Here's how the part is built. I have some questions about the finished solid (model axes, mm). A direction names the side the tool comes from. Give positions to 0.01 mm unless a question says otherwise; leave off trailing zeros. Write each loop counter-clockwise with the first axis right and the second up, starting at its lowest first coordinate (ties: lowest second). Pieces come first, ordered by that corner, then holes. Notation, with made-up numbers: (-9.75, 58) - (46.25, 58) arc R18 ccw to (46.25, 68) - close; hole circle Ø11 at (0, 55.5). An arc over 180 degrees is marked (long way). Use a Markdown table: item, result.
```python
from build123d import *

# Parameters (mm, degrees)
F1_DEPTH = 2
F2_R     = 1
F3_DEPTH = 2.001


with BuildPart() as f1:
    # F0 (on Top) → F1 (new body)
    with BuildSketch(Plane.XY):
        with BuildLine():
            ThreePointArc((7.271564, -1.836943), (7.442672, -0.925546), (7.5, 0))
            ThreePointArc((7.5, 0), (7.442672, 0.925546), (7.271564, 1.836943))
            ThreePointArc((7.271564, 1.836943), (7.132924, 2.317627), (6.962547, 2.788))
            ThreePointArc((6.962547, 2.788), (6.067627, 4.408389), (4.803091, 5.760236))
            ThreePointArc((4.803091, 5.760236), (4.408389, 6.067627), (3.994074, 6.348021))
            ThreePointArc((3.994074, 6.348021), (2.317627, 7.132924), (0.5, 7.483315))
            ThreePointArc((0.5, 7.483315), (0, 7.5), (-0.5, 7.483315))
            ThreePointArc((-0.5, 7.483315), (-2.317627, 7.132924), (-3.994074, 6.348021))
            ThreePointArc((-3.994074, 6.348021), (-4.408389, 6.067627), (-4.803091, 5.760236))
            ThreePointArc((-4.803091, 5.760236), (-6.067627, 4.408389), (-6.962547, 2.788))
            ThreePointArc((-6.962547, 2.788), (-7.132924, 2.317627), (-7.271564, 1.836943))
            ThreePointArc((-7.271564, 1.836943), (-7.5, 0), (-7.271564, -1.836943))
            ThreePointArc((-7.271564, -1.836943), (-7.132924, -2.317627), (-6.962547, -2.788))
            ThreePointArc((-6.962547, -2.788), (-6.067627, -4.408389), (-4.803091, -5.760236))
            ThreePointArc((-4.803091, -5.760236), (-4.408389, -6.067627), (-3.994074, -6.348021))
            ThreePointArc((-3.994074, -6.348021), (-2.317627, -7.132924), (-0.5, -7.483315))
            ThreePointArc((-0.5, -7.483315), (0, -7.5), (0.5, -7.483315))
            ThreePointArc((0.5, -7.483315), (2.317627, -7.132924), (3.994074, -6.348021))
            ThreePointArc((3.994074, -6.348021), (4.408389, -6.067627), (4.803091, -5.760236))
            ThreePointArc((4.803091, -5.760236), (6.067627, -4.408389), (6.962547, -2.788))
            ThreePointArc((6.962547, -2.788), (7.132924, -2.317627), (7.271564, -1.836943))
        make_face()
        with BuildLine():
            ThreePointArc((6.962547, 2.788), (7.132924, 2.317627), (7.271564, 1.836943))
            Line((7.271564, 1.836943), (9.189545, 2.460133))
            Line((9.189545, 2.460133), (9.035037, 2.935661))
            Line((9.035037, 2.935661), (8.880528, 3.41119))
            Line((8.880528, 3.41119), (6.962547, 2.788))
        make_face()
        with BuildLine():
            Line((9.189545, -2.460133), (7.271564, -1.836943))
            ThreePointArc((7.271564, -1.836943), (7.132924, -2.317627), (6.962547, -2.788))
            Line((6.962547, -2.788), (8.880528, -3.41119))
            Line((8.880528, -3.41119), (9.035037, -2.935661))
            Line((9.035037, -2.935661), (9.189545, -2.460133))
        make_face()
        with BuildLine():
            ThreePointArc((3.994074, 6.348021), (4.408389, 6.067627), (4.803091, 5.760236))
            Line((4.803091, 5.760236), (5.988468, 7.391769))
            Line((5.988468, 7.391769), (5.58396, 7.685661))
            Line((5.58396, 7.685661), (5.179451, 7.979554))
            Line((5.179451, 7.979554), (3.994074, 6.348021))
        make_face()
        with BuildLine():
            Line((5.988468, -7.391769), (4.803091, -5.760236))
            ThreePointArc((4.803091, -5.760236), (4.408389, -6.067627), (3.994074, -6.348021))
            Line((3.994074, -6.348021), (5.179451, -7.979554))
            Line((5.179451, -7.979554), (5.58396, -7.685661))
            Line((5.58396, -7.685661), (5.988468, -7.391769))
        make_face()
        with BuildLine():
            ThreePointArc((-0.5, 7.483315), (0, 7.5), (0.5, 7.483315))
            Line((0.5, 7.483315), (0.5, 9.5))
            Line((0.5, 9.5), (0, 9.5))
            Line((0, 9.5), (-0.5, 9.5))
            Line((-0.5, 9.5), (-0.5, 7.483315))
        make_face()
        with BuildLine():
            Line((0.5, -9.5), (0.5, -7.483315))
            ThreePointArc((0.5, -7.483315), (0, -7.5), (-0.5, -7.483315))
            Line((-0.5, -7.483315), (-0.5, -9.5))
            Line((-0.5, -9.5), (0, -9.5))
            Line((0, -9.5), (0.5, -9.5))
        make_face()
        with BuildLine():
            ThreePointArc((-4.803091, 5.760236), (-4.408389, 6.067627), (-3.994074, 6.348021))
            Line((-3.994074, 6.348021), (-5.179451, 7.979554))
            Line((-5.179451, 7.979554), (-5.58396, 7.685661))
            Line((-5.58396, 7.685661), (-5.988468, 7.391769))
            Line((-5.988468, 7.391769), (-4.803091, 5.760236))
        make_face()
        with BuildLine():
            Line((-5.179451, -7.979554), (-3.994074, -6.348021))
            ThreePointArc((-3.994074, -6.348021), (-4.408389, -6.067627), (-4.803091, -5.760236))
            Line((-4.803091, -5.760236), (-5.988468, -7.391769))
            Line((-5.988468, -7.391769), (-5.58396, -7.685661))
            Line((-5.58396, -7.685661), (-5.179451, -7.979554))
        make_face()
        with BuildLine():
            ThreePointArc((-7.271564, 1.836943), (-7.132924, 2.317627), (-6.962547, 2.788))
            Line((-6.962547, 2.788), (-8.880528, 3.41119))
            Line((-8.880528, 3.41119), (-9.035037, 2.935661))
            Line((-9.035037, 2.935661), (-9.189545, 2.460133))
            Line((-9.189545, 2.460133), (-7.271564, 1.836943))
        make_face()
        with BuildLine():
            Line((-8.880528, -3.41119), (-6.962547, -2.788))
            ThreePointArc((-6.962547, -2.788), (-7.132924, -2.317627), (-7.271564, -1.836943))
            Line((-7.271564, -1.836943), (-9.189545, -2.460133))
            Line((-9.189545, -2.460133), (-9.035037, -2.935661))
            Line((-9.035037, -2.935661), (-8.880528, -3.41119))
        make_face()
    extrude(amount=F1_DEPTH)

    # F2 (on face) → F3 (cut, through all)
    with BuildSketch(Plane.XY.offset(2)):
        Circle(F2_R)
    extrude(amount=-F3_DEPTH, mode=Mode.SUBTRACT)


solid = f1.part
```
Item 1: Thinking about a two-plate mould opening in Y: for faces 4 (the flat face through (5.387, 6.565, 0.986)), 5 (the flat face through (-0.5, -8, 1)), 6 (the flat face through (5.404, -6.587, 0.986)), 7 (the cylindrical face through (2.29, -7.14, 0.99)), which applies, +Y half, -Y half, draft (parallel to the pull), parting line (faces both ways), or undercut?
Values:
| item | result |
|---|---|
| face 4 | undercut |
| face 5 | draft |
| face 6 | undercut |
| face 7 | -Y half |
Item 2: Will this pin go through, and if not, where does the flat tip stop? pin 1 Ø1 at (y, z) = (8, 1) entering from -X.
Values:
| item | result |
|---|---|
| pin 1 | stops at x = -5.84 |
Item 3: If we section it at C-C, the plane x = -6.5: Write out the boundary of the cut face in (y, z).
Values:
| item | result |
|---|---|
| outline | (-3.74, 0) - (3.74, 0) - (3.74, 2) - (-3.74, 2) - close |
Item 4: I need wall thicknesses on line 1 along Y through (x, z) = (0, 0.6); line 2 along Y through (x, z) = (5.75, 0.55); line 3 along X through (y, z) = (-7.75, 0.2). Which ranges of each line are inside material? Lowest first, please. Write a range as [from, to].
Values:
| item | result |
|---|---|
| line 1 | y = [-9.5, -1], [1, 9.5] |
| line 2 | y = [-7.57, -7.06], [-4.82, 4.82], [7.06, 7.57] |
| line 3 | x = [-5.5, -5.01], [-0.5, 0.5], [5.01, 5.5] |
Item 5: If we section it at B-B, the plane y = 1.5: Write out the boundary of the cut face in (x, z).
Values:
| item | result |
|---|---|
| outline | (-7.35, 0) - (7.35, 0) - (7.35, 2) - (-7.35, 2) - close |
Item 6: If we section it at A-A, the plane x = 0: Write out the boundary of the cut face in (y, z), plus the area to 3 significant figures.
Values:
| item | result |
|---|---|
| outline | (-9.5, 0) - (-1, 0) - (-1, 2) - (-9.5, 2) - close; (1, 0) - (9.5, 0) - (9.5, 2) - (1, 2) - close |
| area | 34.0 mm2 |
Item 7: For faces 1 (the cylindrical face through (-6.05, 4.43, 0.99)), 2 (the flat face through (-5.404, 6.587, 0.986)), 3 (the flat face through (0.5, 8, 1)), which set-ups out of +Z, -Z, +X, -X, +Y, -Y let a thin tool reach every point of the face, with its end or its side?
Values:
| item | result |
|---|---|
| face 1 | +Z, -Z |
| face 2 | +Z, -Z, -X |
| face 3 | +Z, -Z, +Y |
